Input: dimensioned drawing with shaded views. Units: mm. Origin: part minimum x, y, z. Round coordinates to 2 decimals unless told otherwise and drop trailing zeros. Loops run counter-clockwise (first coordinate to the right, second up) from the corner with the lowest first, then second, coordinate; pieces in that order, holes last. Notation, with made-up numbers: M 63,82 L 92,82 A23 ccw 92,100 Z; hole C -13,-28.5 d1. An arc over 180 degrees is marked long. Write each question's results on one line, items separated by ' | '. Start each with the question number.
1. Section B-B on x = 27.5. Output: boundary loops of the cut face in (y, z).
2. Section C-C on y = 0.6. Give the number of separate pieces and of enclosed holes in the cut face, and give its area (3 significant figures).
3. Section A-A on z = 7.5. Output: boundary loops of the cut face in (x, y).
4. Ray query, line 1 (Z direction, x = 27.5, y = 1); line 2 (X direction, y = 1.15, z = 7.5); line 3 (X direction, y = 1.6, z = 94). Return the intervals inside material, ascending.
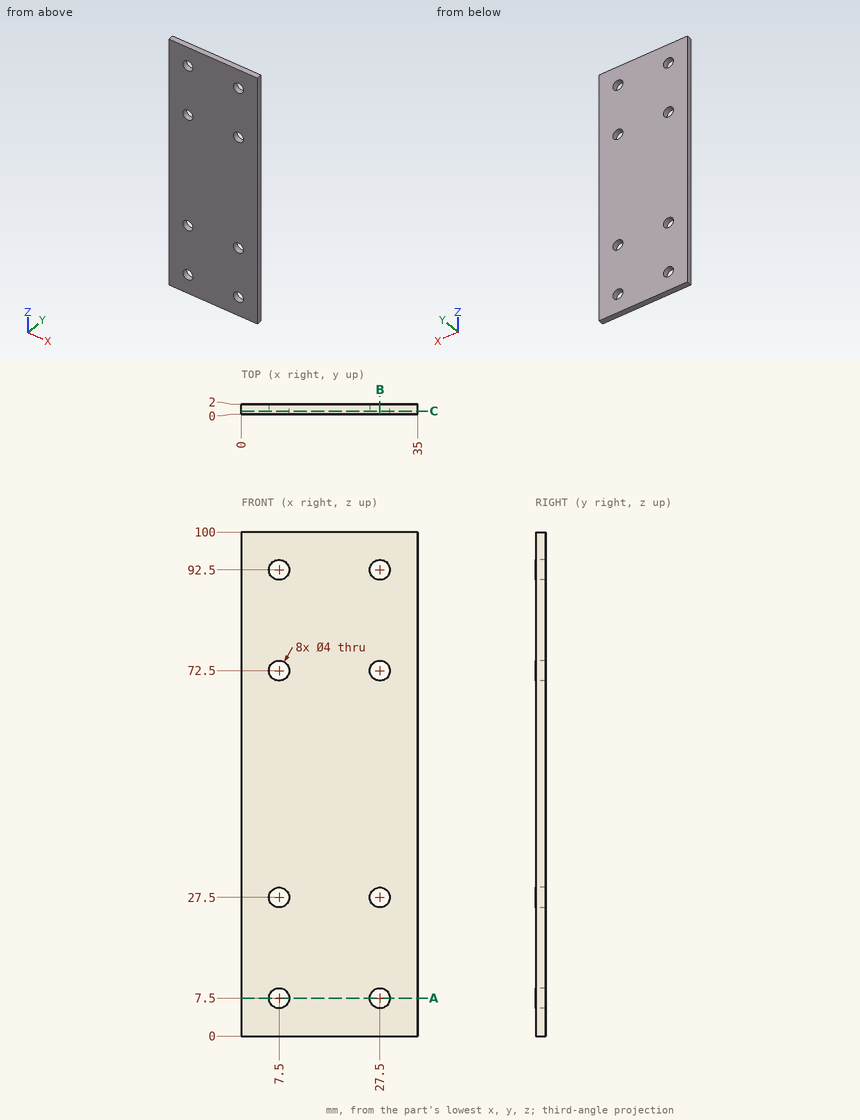
Taken from the geometry:
1) outline: M 0,0 L 2,0 L 2,5.5 L 0,5.5 Z; M 0,9.5 L 2,9.5 L 2,25.5 L 0,25.5 Z; M 0,29.5 L 2,29.5 L 2,70.5 L 0,70.5 Z; M 0,74.5 L 2,74.5 L 2,90.5 L 0,90.5 Z; M 0,94.5 L 2,94.5 L 2,100 L 0,100 Z
2) separate pieces: 1 | enclosed holes: 8 | area: 3,400 mm^2
3) outline: M 0,0 L 5.5,0 L 5.5,2 L 0,2 Z; M 9.5,0 L 25.5,0 L 25.5,2 L 9.5,2 Z; M 29.5,0 L 35,0 L 35,2 L 29.5,2 Z
4) line 1: 0 to 5.5, 9.5 to 25.5, 29.5 to 70.5, 74.5 to 90.5, 94.5 to 100 | line 2: 0 to 5.5, 9.5 to 25.5, 29.5 to 35 | line 3: 0 to 6.18, 8.82 to 26.18, 28.82 to 35
